Part print with two shaded views. Sizes in mm from the minimum x, y, z corner. Give positions to 0.01 mm unless a question says otherwise; leave off trailing zeros. Write each loop counter-clockwise with the first axis right and the second up, starting at its lowest first coordinate (ties: lowest second). Pieces come first, ordered by that corner, then holes. Notation, with made-up numbers: (70.5, 43.25) - (114.5, 43.25) arc R17 ccw to (114.5, 60.25) - close; hole circle Ø1 at (57, 65.5). An arc over 180 degrees is marked (long way). Answer as a JSON object with one key per item and string values.
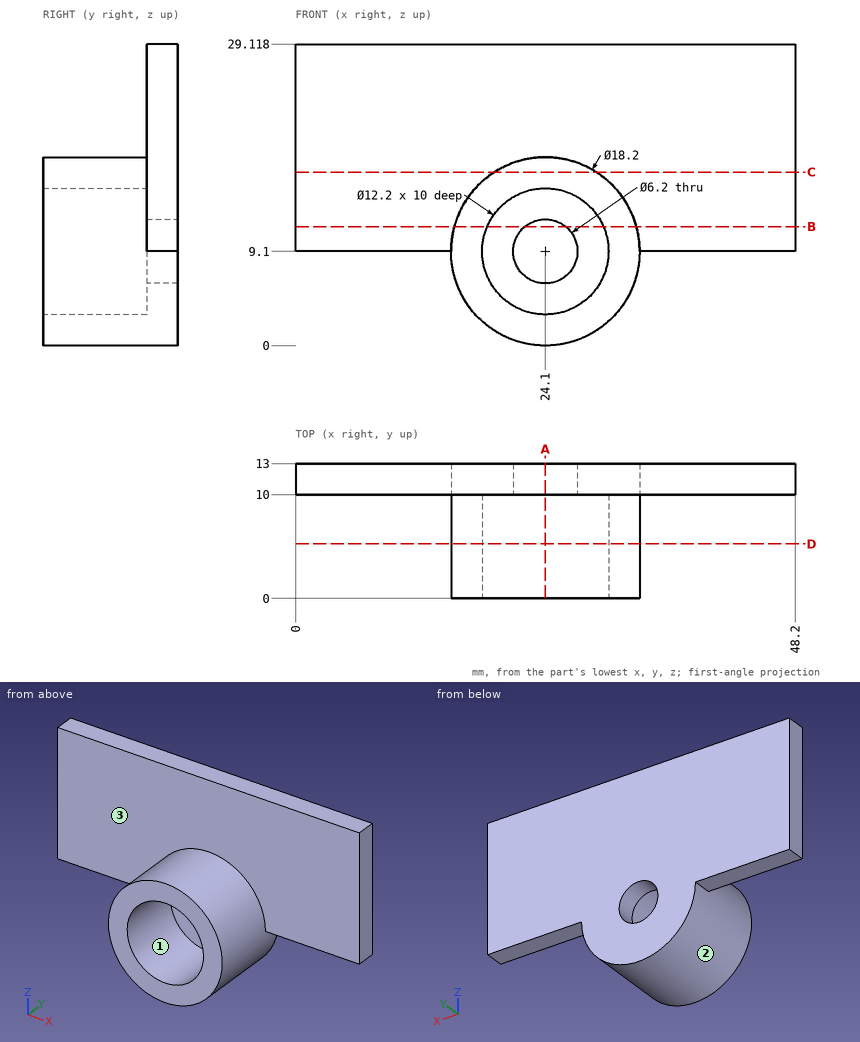
(1) Flat gauge pins, fed straight in: P1, Ø3.5, axis at x = 4.5, y = 12, coming from the -Z side; P2, Ø3, axis at x = 14, z = 15.5, coming from the -Y side; P3, Ø8, axis at x = 21.5, z = 8, coming from the -Y side; P4, Ø2, axis at x = 21.5, y = 7, coming from the -Z side. Where does each tip first touch, or does it go through?
Answer key:
{"P1": "stops at z = 9.1", "P2": "stops at y = 10", "P3": "stops at y = 0", "P4": "stops at z = 0.14"}
(2) Saw through at B-B, the plane z = 11.5. Give the cut face in (x, y), and give its area (3 significant figures).
Answer key:
{"outline": "(0, 10) - (15.32, 10) - (15.32, 0) - (18.49, 0) - (18.49, 10) - (22.14, 10) - (22.14, 13) - (0, 13) - close; (26.06, 10) - (29.71, 10) - (29.71, 0) - (32.88, 0) - (32.88, 10) - (48.2, 10) - (48.2, 13) - (26.06, 13) - close", "area": "196 mm²"}
(3) Pull direction Z, two halves, no side cores. Call the marked faces 1, 2 and 3: pulls with the +Z half, pulls with the -Z half, needs draft (parallel to the pull), parting line crosses it, or undercut.
Answer key:
{"face 1": "undercut", "face 2": "parting line crosses it", "face 3": "needs draft"}
(4) Probe L1, parallel to X at y = 2, z = 9.1; L2, parallel to Y at x = 27.5, z = 5.5; L3, parallel to X at y = 3.25, z = 7 (1 decimal). List the from-to ranges inside material, lowest first. Write a range as [from, to].
Answer key:
{"L1": "x = [15, 18], [30.2, 33.2]", "L2": "y = [10, 13]", "L3": "x = [15.2, 18.4], [29.8, 33]"}
(5) Saw through at C-C, the plane z = 16.75. Give the cut face in (x, y), and give its area (3 significant figures).
Answer key:
{"outline": "(0, 10) - (19.17, 10) - (19.17, 0) - (29.03, 0) - (29.03, 10) - (48.2, 10) - (48.2, 13) - (0, 13) - close", "area": "243 mm²"}
(6) Saw through at D-D, the plane y = 5.25. Give the cut face in (x, z).
Answer key:
{"outline": "circle Ø18.2 at (24.1, 9.1); hole circle Ø12.2 at (24.1, 9.1)"}
(7) Saw through at A-A, the plane x = 24.1. Give the cut face in (y, z), and give its area (3 significant figures).
Answer key:
{"outline": "(0, 0) - (13, 0) - (13, 6) - (10, 6) - (10, 3) - (0, 3) - close; (0, 15.2) - (10, 15.2) - (10, 12.2) - (13, 12.2) - (13, 29.12) - (10, 29.12) - (10, 18.2) - (0, 18.2) - close", "area": "129 mm²"}
